from build123d import *

# Parameters (mm, degrees)
ESQUISSE1_R                   = 1.15
ESQUISSE1_R_2                 = 1.75
ESQUISSE1_R_3                 = 1
ESQUISSE1_W                   = 18
ESQUISSE1_H                   = 33.5
BOSS_EXTRU_2_DEPTH            = 12
ENL_V_MAT_EXTRU_1_DEPTH       = 75.057589753
ESQUISSE3_W                   = 2.3
ESQUISSE3_H                   = 33.5
ESQUISSE3_W_2                 = 2
ESQUISSE3_H_2                 = 16
ENL_V_MAT_EXTRU_2_DEPTH       = 74.753146373
CONG_1_R                      = 3
ENL_V_MAT_EXTRU_3_REACH       = 62.317
ESQUISSE4_R                   = 2.2
ENL_V_MAT_EXTRU_4_REACH       = 67.556
ESQUISSE5_R                   = 3.5
ESQUISSE6_R                   = 3.5
ENL_V_MAT_EXTRU_5_DEPTH       = 5
ESQUISSE7_W                   = 8.040923999
ESQUISSE7_H                   = 1.8
ENL_V_MAT_EXTRU_6_DEPTH       = 1
ENL_V_MAT_EXTRU_7_DEPTH       = 3
ENL_V_MAT_EXTRU_7_DEPTH_BACK  = 75.185757393
ESQUISSE8_W                   = 24.177827552
ESQUISSE8_H                   = 3.5
ENL_V_MAT_EXTRU_8_REACH       = 72.034
ENL_V_MAT_EXTRU_9_REACH       = 76.033
ESQUISSE10_R                  = 4
ESQUISSE11_R                  = 12.099999999
ENL_V_MAT_EXTRU_10_DEPTH      = 76.583950893
ENL_V_MAT_EXTRU_11_DEPTH      = 38
ENL_V_MAT_EXTRU_11_DEPTH_BACK = 1
ESQUISSE17_R                  = 1.5
ENL_V_MAT_EXTRU_12_DEPTH      = 13
ENL_V_MAT_EXTRU_12_DEPTH_BACK = 1.2
ESQUISSE18_R                  = 1.5


with BuildPart() as part:
    # Esquisse1 → Boss.-Extru.2 (new body)
    with BuildSketch(Plane.XY):
        with BuildLine():
            Line((-12.306087575, 57.58118588), (-12.306087575, 54.58118588))
            Line((-12.306087575, 54.58118588), (12.393912425, 33.78118588))
            Line((12.393912425, 33.78118588), (19.393912425, 33.78118588))
            Line((19.393912425, 33.78118588), (20.993912425, 29.58118588))
            Line((20.993912425, 29.58118588), (45.693912425, 29.58118588))
            Line((45.693912425, 29.58118588), (45.693912425, -1.41881412))
            Line((45.693912425, -1.41881412), (18.993912425, -1.41881412))
            Line((18.993912425, -1.41881412), (18.993912425, -16.91881412))
            Line((18.993912425, -16.91881412), (8.993912425, -16.91881412))
            Line((8.993912425, -16.91881412), (8.993912425, -15.66881412))
            Line((8.993912425, -15.66881412), (-1.006087575, -15.66881412))
            Line((-1.006087575, -15.66881412), (-1.006087575, -16.91881412))
            Line((-1.006087575, -16.91881412), (-9.006087575, -16.91881412))
            Line((-9.006087575, -16.91881412), (-9.006087575, -15.66881412))
            Line((-9.006087575, -15.66881412), (-13.006087575, -15.66881412))
            Line((-13.006087575, -15.66881412), (-13.006087575, -11.91881412))
            Line((-13.006087575, -11.91881412), (-13.676087575, -11.91881412))
            ThreePointArc((-13.676087575, -11.91881412), (-16.030753157, -10.943479702), (-17.006087575, -8.58881412))
            Line((-17.006087575, -8.58881412), (-17.006087575, 57.58118588))
            Line((-17.006087575, 57.58118588), (-12.306087575, 57.58118588))
        make_face()
        with Locations((-13.676087575, -8.58881412)):
            Circle(ESQUISSE1_R, mode=Mode.SUBTRACT)
        with Locations((-13.676087575, 20.41118588)):
            Circle(ESQUISSE1_R_2, mode=Mode.SUBTRACT)
        with Locations((15.323912425, -13.41881412)):
            Circle(ESQUISSE1_R_2, mode=Mode.SUBTRACT)
        with Locations((38.693912425, 5.58118588)):
            Circle(ESQUISSE1_R_2, mode=Mode.SUBTRACT)
        with Locations((23.193912425, 3.58118588)):
            Circle(ESQUISSE1_R_3, mode=Mode.SUBTRACT)
        with Locations((23.193912425, 20.58118588)):
            Circle(ESQUISSE1_R_3, mode=Mode.SUBTRACT)
        with Locations((14.693912425, 29.08118588)):
            Circle(ESQUISSE1_R_3, mode=Mode.SUBTRACT)
        with Locations((-2.006087575, 1.83118588)):
            Rectangle(ESQUISSE1_W, ESQUISSE1_H, mode=Mode.SUBTRACT)
    extrude(amount=BOSS_EXTRU_2_DEPTH)

    # Esquisse2 → Enlèv. mat.-Extru.1 (cut, through all)
    # profile 1 of 4: a face of its own
    with BuildSketch(Plane.XY.offset(9)):
        with BuildLine():
            ThreePointArc((25.047962046, 19.83118588), (23.193912425, 22.58118588), (21.339862803, 19.83118588))
            Line((21.339862803, 19.83118588), (11.493912425, 19.83118588))
            Line((11.493912425, 19.83118588), (11.493912425, 20.58118588))
            Line((11.493912425, 20.58118588), (-10.010027019, 20.58118588))
            ThreePointArc((-10.010027019, 20.58118588), (-11.141822396, 23.065691483), (-13.676087575, 24.08118588))
            Line((-13.676087575, 24.08118588), (-14.706087575, 24.08118588))
            Line((-14.706087575, 24.08118588), (-14.706087575, 57.58118588))
            Line((-14.706087575, 57.58118588), (-12.306087575, 57.58118588))
            Line((-12.306087575, 57.58118588), (-12.306087575, 54.58118588))
            Line((-12.306087575, 54.58118588), (12.393912425, 33.78118588))
            Line((12.393912425, 33.78118588), (19.393912425, 33.78118588))
            Line((19.393912425, 33.78118588), (20.993912425, 29.58118588))
            Line((20.993912425, 29.58118588), (43.693912425, 29.58118588))
            Line((43.693912425, 29.58118588), (43.693912425, 6.58118588))
            Line((43.693912425, 6.58118588), (42.048014391, 6.58118588))
            ThreePointArc((42.048014391, 6.58118588), (38.693912425, 9.08118588), (35.339810458, 6.58118588))
            Line((35.339810458, 6.58118588), (26.693912425, 6.58118588))
            Line((26.693912425, 6.58118588), (26.693912425, 5.88118588))
            Line((26.693912425, 5.88118588), (6.993912425, 5.88118588))
            Line((6.993912425, 5.88118588), (6.993912425, 15.83118588))
            Line((6.993912425, 15.83118588), (11.493912425, 15.83118588))
            Line((11.493912425, 15.83118588), (11.493912425, 17.83118588))
            Line((11.493912425, 17.83118588), (31.493912425, 17.83118588))
            Line((31.493912425, 17.83118588), (31.493912425, 19.83118588))
            Line((31.493912425, 19.83118588), (25.047962046, 19.83118588))
        make_face()
        with BuildLine():
            ThreePointArc((16.616800877, 28.53118588), (14.693912425, 31.08118588), (12.771023972, 28.53118588))
            Line((12.771023972, 28.53118588), (-2.006087575, 28.53118588))
            Line((-2.006087575, 28.53118588), (-2.006087575, 26.83118588))
            Line((-2.006087575, 26.83118588), (18.993912425, 26.83118588))
            Line((18.993912425, 26.83118588), (18.993912425, 28.53118588))
            Line((18.993912425, 28.53118588), (16.616800877, 28.53118588))
        make_face(mode=Mode.SUBTRACT)
    # profile 2 of 4: a face of its own
    with BuildSketch(Plane.XY.offset(9)):
        with BuildLine():
            ThreePointArc((20.964002112, 3.88118588), (21.206819115, 2.52574276), (22.193912425, 1.565621443))
            Line((22.193912425, 1.565621443), (22.193912425, 0.58118588))
            Line((22.193912425, 0.58118588), (18.993912425, 0.58118588))
            Line((18.993912425, 0.58118588), (18.993912425, -9.51881412))
            Line((18.993912425, -9.51881412), (9.993912425, -9.51881412))
            Line((9.993912425, -9.51881412), (9.993912425, -14.91881412))
            Line((9.993912425, -14.91881412), (6.993912425, -14.91881412))
            Line((6.993912425, -14.91881412), (6.993912425, 3.88118588))
            Line((6.993912425, 3.88118588), (20.964002112, 3.88118588))
        make_face()
    # profile 3 of 4: a face of its own
    with BuildSketch(Plane.XY.offset(9)):
        with BuildLine():
            ThreePointArc((-15.006087575, 17.173733177), (-12.847657165, 17.010641356), (-11.006087575, 18.148201125))
            Line((-11.006087575, 18.148201125), (-11.006087575, -7.220932547))
            ThreePointArc((-11.006087575, -7.220932547), (-12.735191712, -5.740180242), (-15.006087575, -5.899743649))
            Line((-15.006087575, -5.899743649), (-15.006087575, 17.173733177))
        make_face()
    # profile 4 of 4: a face of its own
    with BuildSketch(Plane.XY.offset(9)):
        with BuildLine():
            ThreePointArc((24.193912425, 1.565621443), (25.181005734, 2.52574276), (25.423822737, 3.88118588))
            Line((25.423822737, 3.88118588), (29.193912425, 3.88118588))
            Line((29.193912425, 3.88118588), (29.193912425, 4.58118588))
            Line((29.193912425, 4.58118588), (35.339810458, 4.58118588))
            ThreePointArc((35.339810458, 4.58118588), (38.693912425, 2.08118588), (42.048014391, 4.58118588))
            Line((42.048014391, 4.58118588), (43.693912425, 4.58118588))
            Line((43.693912425, 4.58118588), (43.693912425, 0.58118588))
            Line((43.693912425, 0.58118588), (24.193912425, 0.58118588))
            Line((24.193912425, 0.58118588), (24.193912425, 1.565621443))
        make_face()
    extrude(amount=-ENL_V_MAT_EXTRU_1_DEPTH, mode=Mode.SUBTRACT)

    # Esquisse3 → Enlèv. mat.-Extru.2 (cut, through all)
    with BuildSketch(Plane.XY.offset(6)):
        with Locations((-15.856087575, 40.83118588)):
            Rectangle(ESQUISSE3_W, ESQUISSE3_H)
        with Locations((44.693912425, 21.58118588)):
            Rectangle(ESQUISSE3_W_2, ESQUISSE3_H_2)
    extrude(amount=-ENL_V_MAT_EXTRU_2_DEPTH, mode=Mode.SUBTRACT)

    # Congé1
    cong_1_edges = [part.edges().sort_by_distance(p)[0] for p in [
        (9.993912425, -9.51881412, 4.5),
    ]]
    fillet(cong_1_edges, radius=CONG_1_R)

    # Esquisse4 → Enlèv. mat.-Extru.3 (cut, up to next)
    with BuildSketch(Plane(origin=(0, 20.58118588, 0), x_dir=(1, 0, 0), z_dir=(0, 1, 0)), mode=Mode.PRIVATE) as enl_v_mat_extru_3_sk1:
        with Locations((-2.006087575, 0)):
            Circle(ESQUISSE4_R)
    enl_v_mat_extru_3_tool1 = extrude(enl_v_mat_extru_3_sk1.sketch, amount=-ENL_V_MAT_EXTRU_3_REACH, mode=Mode.PRIVATE) & part.part
    add(enl_v_mat_extru_3_tool1.solids().sort_by_distance((-2.006088, 20.581186, 0))[0], mode=Mode.SUBTRACT)

    # Esquisse5 → Enlèv. mat.-Extru.4 (cut, up to next)
    with BuildSketch(Plane(origin=(0, 28.53118588, 0), x_dir=(1, 0, 0), z_dir=(0, 1, 0)), mode=Mode.PRIVATE) as enl_v_mat_extru_4_sk1:
        with Locations((-2.017786304, -0.014313461)):
            Circle(ESQUISSE5_R)
    enl_v_mat_extru_4_tool1 = extrude(enl_v_mat_extru_4_sk1.sketch, amount=-ENL_V_MAT_EXTRU_4_REACH, mode=Mode.PRIVATE) & part.part
    add(enl_v_mat_extru_4_tool1.solids().sort_by_distance((-2.017786, 28.531186, 0.014313))[0], mode=Mode.SUBTRACT)

    # Esquisse6 → Enlèv. mat.-Extru.5 (cut)
    with BuildSketch(Plane(origin=(0, 19.83118588, 0), x_dir=(1, 0, 0), z_dir=(0, 1, 0))):
        with Locations((14.993912425, 0)):
            Circle(ESQUISSE6_R)
    extrude(amount=-ENL_V_MAT_EXTRU_5_DEPTH, mode=Mode.SUBTRACT)

    # Esquisse7 → Enlèv. mat.-Extru.6 (cut)
    with BuildSketch(Plane(origin=(0, 0, 9), x_dir=(-1, 0, 0), z_dir=(0, 0, -1))):
        with Locations((2.077482888, 31.18118588)):
            Rectangle(ESQUISSE7_W, ESQUISSE7_H)
    extrude(amount=-ENL_V_MAT_EXTRU_6_DEPTH, mode=Mode.SUBTRACT)

    # Esquisse8 → Enlèv. mat.-Extru.7 (cut, two sides: drawn at the far end of the back side and taken through both)
    with BuildSketch(Plane(origin=(0, 0, 10), x_dir=(-1, 0, 0), z_dir=(0, 0, -1)).offset(-ENL_V_MAT_EXTRU_7_DEPTH_BACK)):
        with Locations((-14.607691418, 24.992571009)):
            Rectangle(ESQUISSE8_W, ESQUISSE8_H)
    extrude(amount=ENL_V_MAT_EXTRU_7_DEPTH + ENL_V_MAT_EXTRU_7_DEPTH_BACK, mode=Mode.SUBTRACT)

    # Esquisse9 → Enlèv. mat.-Extru.8 (cut, up to next)
    with BuildSketch(Plane(origin=(0, 5.88118588, 0), x_dir=(1, 0, 0), z_dir=(0, 1, 0)), mode=Mode.PRIVATE) as enl_v_mat_extru_8_sk1:
        with BuildLine():
            Line((19.993912425, 0), (6.993912425, 0))
            Line((6.993912425, 0), (6.993912425, -5))
            Line((6.993912425, -5), (14.993912425, -5))
            ThreePointArc((14.993912425, -5), (18.529446331, -3.535533906), (19.993912425, 0))
        make_face()
    enl_v_mat_extru_8_tool1 = extrude(enl_v_mat_extru_8_sk1.sketch, amount=-ENL_V_MAT_EXTRU_8_REACH, mode=Mode.PRIVATE) & part.part
    add(enl_v_mat_extru_8_tool1.solids().sort_by_distance((13.009618, 5.881186, 2.375564))[0], mode=Mode.SUBTRACT)

    # Esquisse10 → Enlèv. mat.-Extru.9 (cut, up to next)
    with BuildSketch(Plane(origin=(0, 0.58118588, 0), x_dir=(1, 0, 0), z_dir=(0, 1, 0)), mode=Mode.PRIVATE) as enl_v_mat_extru_9_sk1:
        with Locations((29.993541661, 0.105464602)):
            Circle(ESQUISSE10_R)
    enl_v_mat_extru_9_tool1 = extrude(enl_v_mat_extru_9_sk1.sketch, amount=-ENL_V_MAT_EXTRU_9_REACH, mode=Mode.PRIVATE) & part.part
    add(enl_v_mat_extru_9_tool1.solids().sort_by_distance((29.993542, 0.581186, -0.105465))[0], mode=Mode.SUBTRACT)

    # Esquisse11 → Enlèv. mat.-Extru.10 (cut, through all)
    with BuildSketch(Plane.XZ.offset(1.41881412)):
        with Locations((29.993541661, -0.105464602)):
            Circle(ESQUISSE11_R)
    extrude(amount=ENL_V_MAT_EXTRU_10_DEPTH, mode=Mode.SUBTRACT)

    # Esquisse17 → Enlèv. mat.-Extru.11 (cut, two sides: drawn at the far end of the back side and taken through both)
    with BuildSketch(Plane.XZ.offset(-26.83118588).offset(-ENL_V_MAT_EXTRU_11_DEPTH_BACK)):
        with Locations((14.993912425, 0)):
            Circle(ESQUISSE17_R)
    extrude(amount=ENL_V_MAT_EXTRU_11_DEPTH + ENL_V_MAT_EXTRU_11_DEPTH_BACK, mode=Mode.SUBTRACT)

    # Esquisse18 → Enlèv. mat.-Extru.12 (cut, two sides: drawn at the far end of the back side and taken through both)
    with BuildSketch(Plane.XZ.offset(-17.83118588).offset(-ENL_V_MAT_EXTRU_12_DEPTH_BACK)):
        with Locations((23.993912425, 0)):
            Circle(ESQUISSE18_R)
    extrude(amount=ENL_V_MAT_EXTRU_12_DEPTH + ENL_V_MAT_EXTRU_12_DEPTH_BACK, mode=Mode.SUBTRACT)


solid = part.part
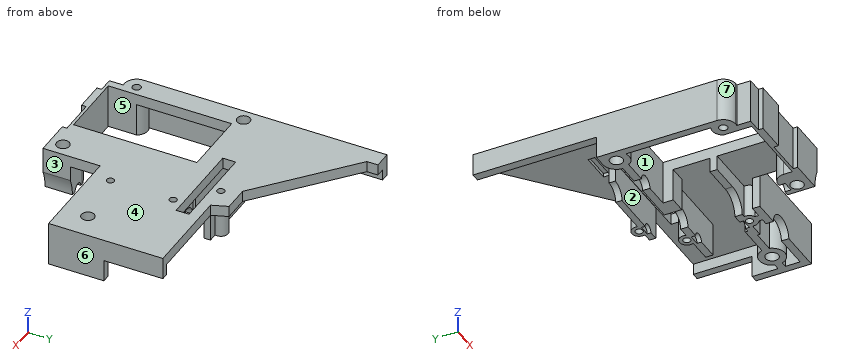
Could you check a few things on this model? Use its own coordinates, in mm. Face numbers are marked on the shaded views. A direction names the side the tool comes from. Give positions to 0.01 mm unless a question says otherwise; leave off trailing zeros. Order: outer loops, then holes, each group sorted by start corner. A loop starts at its lowest first (then second) coordinate and runs counter-clockwise, first axis right, second up. Notation, with made-up numbers: (85.5, -38.5) - (144.5, -38.5) arc R21 ccw to (144.5, -8.5) - close; hole circle Ø8 at (66.25, -31). An arc over 180 degrees is marked (long way). Return JSON: item names as keys, results as strings. Group by question number.
Q1. Suppose I cut it at A-A, the plane y = 12.5. Please give me the cut outline in (x, z).
Q2. Thinking about a two-plate mould opening in X: for the marked faces 5, 6 and 7, which applies, pulls with the +X half, pulls with the -X half, needs draft (parallel to the pull), parting line crosses it, or undercut?
Q3. Please list where these lines run through material, in increasing order: line 1 along Y through (x, z) = (4, 4); line 2 along X through (y, z) = (20.5, 5.75); line 3 along Y through (x, z) = (-3, 9.5). Write a range as [from, to].
Q4. Suppose I cut it at B-B, the plane x = 5.5. Please give me the cut outline in (y, z), and give its area (3 significant figures).
Q5. Which directions (+Z, -Z, +X, -X, +Y, -Y) give clear straight access to the entire face, cutting with the end or side of a thin tool? Please do the marked faces 1, 2, 3 and 4.
Q6. Will these pins go through, and if not, where does the flat tip stop? pin 1 Ø3 at (x, z) = (27, 3.5) entering from +Y; pin 2 Ø0.8 at (y, z) = (31.5, 9.5) entering from +X; pin 3 Ø1.5 at (x, y) = (6.5, 30.5) entering from -Z.
Resolved:
{
 "1": {"outline": "(-17.01, 0) - (-15.01, 0) - (-15.01, 9) - (-11.01, 9) - (-11.01, 12) - (-17.01, 12) - close; (6.99, 9) - (43.69, 9) - (43.69, 0) - (45.69, 0) - (45.69, 12) - (6.99, 12) - close"},
 "2": {"face 5": "undercut", "face 6": "pulls with the +X half", "face 7": "pulls with the -X half"},
 "3": {"line 1": "y = [-15.67, -14.92], [18.58, 20.58], [26.83, 28.53]", "line 2": "x = [-17.01, -15.42], [-11.93, 11.49], [21.2, 22.2], [24.19, 25.19]", "line 3": "y = [-16.92, -14.92], [18.58, 30.28], [32.08, 46.74]"},
 "4": {"outline": "(-15.67, 0) - (-14.92, 0) - (-14.92, 12) - (-15.67, 12) - close; (18.58, 0) - (20.58, 0) - (20.58, 9) - (23.24, 9) - (23.24, 12) - (18.58, 12) - close; (26.74, 9) - (26.83, 9) - (26.83, 0) - (28.53, 0) - (28.53, 9) - (39.59, 9) - (39.59, 12) - (26.74, 12) - close", "area": "94.8 mm2"},
 "5": {"face 1": "+Z, -Z", "face 2": "-Z", "face 3": "+Z, -Z, +X, -Y", "face 4": "+Z, +X, -X, +Y, -Y"},
 "6": {"pin 1": "stops at y = 19.83", "pin 2": "stops at x = 20.42", "pin 3": "stops at z = 9"}
}
